from build123d import *

# Parameters (mm, degrees)
BOSS_EXTRUDE2_DEPTH = 20
CUT_EXTRUDE1_DEPTH  = 20
CUT_EXTRUDE2_DEPTH  = 20


with BuildPart() as part:
    # Sketch1 → Boss-Extrude2 (new body)
    with BuildSketch(Plane.XY):
        Polygon((0, 0), (17.38, 0), (17.38, 3.4), (3.4, 3.4), (3.4, 21.15), (0, 21.15), align=None)
    extrude(amount=BOSS_EXTRUDE2_DEPTH)

    # Sketch2 → Cut-Extrude1 (cut)
    with BuildSketch(Plane(origin=(3.4, 0, 0), x_dir=(0, 0, -1), z_dir=(1, 0, 0))):
        with BuildLine():
            Line((-7, 13.775), (-7, 10.775))
            ThreePointArc((-7, 10.775), (-10, 7.775), (-13, 10.775))
            Line((-13, 10.775), (-13, 13.775))
            ThreePointArc((-13, 13.775), (-10, 16.775), (-7, 13.775))
        make_face()
    extrude(amount=-CUT_EXTRUDE1_DEPTH, mode=Mode.SUBTRACT)

    # Sketch3 → Cut-Extrude2 (cut)
    with BuildSketch(Plane(origin=(0, 3.4, 0), x_dir=(1, 0, 0), z_dir=(0, 1, 0))):
        with BuildLine():
            Line((8.89, -7), (11.89, -7))
            ThreePointArc((11.89, -7), (14.89, -10), (11.89, -13))
            Line((11.89, -13), (8.89, -13))
            ThreePointArc((8.89, -13), (5.89, -10), (8.89, -7))
        make_face()
    extrude(amount=-CUT_EXTRUDE2_DEPTH, mode=Mode.SUBTRACT)


solid = part.part
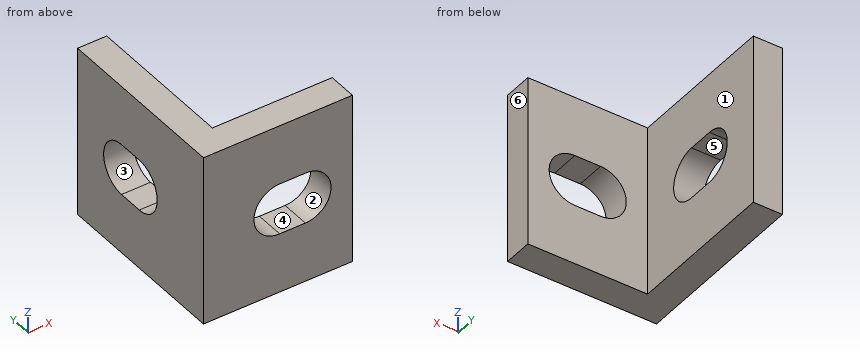
Here's how the part is built. I have some questions about the finished solid (model axes, mm). Face numbers are marked on the shaded views. A direction names the side the tool comes from. Round coordinates to 2 decimals unless told otherwise and drop trailing zeros. Write each loop counter-clockwise with the first axis right and the second up, starting at its lowest first coordinate (ties: lowest second). Pieces come first, ordered by that corner, then holes.
1. Suppose I cut it at B-B (z = 10). List the corners of the cut face in (x, y) for me (3 decimals).
2. Suppose I cut it at A-A (x = 11). List the corners of the cut face in (y, z) for me, and give its area (3 significant figures).
3. If we mould it in two halves opening along X, with no side actions, what happens to the marked faces 4, 5 and 6? For each: released by +X, released by -X, zero draft, split by the parting line, or undercut.
4. Suppose I cut it at C-C (y = 15.75). List the corners of the cut face in (x, z) for me, and give its area (3 significant figures).
5. For the marked faces 1, 2 and 3, which set-ups out of +Z, -Z, +X, -X, +Y, -Y let a thin tool reach every point of the face, with its end or its side?
6. I need wall thicknesses on L1, parallel to Z at x = 11, y = 2.75; L2, parallel to Y at x = 11, z = 1.25. Which ranges of each line are inside material? Lowest first, please.
7. Will these pins go through, and if not, where does the flat tip stop? pin 1 Ø2 at (x, z) = (12, 4.5) entering from -Y; pin 2 Ø1.5 at (y, z) = (10, 7.5) entering from +X; pin 3 Ø2 at (x, z) = (15, 6.5) entering from +Y.
8. Suppose I cut it at D-D (z = 2.5). List the corners of the cut face in (x, y) for me.
Answer sheet:
1. outline: (0, 0) - (5.89, 0) - (5.89, 3.4) - (3.4, 3.4) - (3.4, 7.775) - (0, 7.775) - close; (0, 16.775) - (3.4, 16.775) - (3.4, 21.15) - (0, 21.15) - close; (14.89, 0) - (17.38, 0) - (17.38, 3.4) - (14.89, 3.4) - close
2. outline: (0, 0) - (3.4, 0) - (3.4, 7) - (0, 7) - close; (0, 13) - (3.4, 13) - (3.4, 20) - (0, 20) - close
2. area: 47.6 mm2
3. face 4: undercut
3. face 5: zero draft
3. face 6: released by +X
4. outline: (0, 0) - (3.4, 0) - (3.4, 7.74) - (0, 7.74) - close; (0, 12.26) - (3.4, 12.26) - (3.4, 20) - (0, 20) - close
4. area: 52.6 mm2
5. face 1: +Z, -Z, +X, +Y
5. face 2: +Y, -Y
5. face 3: +X, -X
6. L1: z = 0 to 7, 13 to 20
6. L2: y = 0 to 3.4
7. pin 1: stops at y = 0
7. pin 2: stops at x = 3.4
7. pin 3: stops at y = 3.4
8. outline: (0, 0) - (17.38, 0) - (17.38, 3.4) - (3.4, 3.4) - (3.4, 21.15) - (0, 21.15) - close
